Geometry: final body of the model. Coordinates: model frame, mm. Give positions to 0.01 mm unless a question says otherwise; leave off trailing zeros. Loops run counter-clockwise (first coordinate to the right, second up) from the corner with the lowest first, then second, coordinate; pieces in that order, holes last. Notation, with made-up numbers: (-39.75, 8.5) - (14.25, 8.5) arc R25 ccw to (14.25, 45.5) - close; hole circle Ø1 at (43.25, 5.5). An arc over 180 degrees is marked (long way). Answer in a Markdown table with one row per item.
from build123d import *

# Parameters (mm, degrees)
SKETCH_1_W      = 110
SKETCH_1_H      = 116
SKETCH_1_R      = 4.5
SKETCH_1_R_2    = 2
EXTRUDE_1_DEPTH = 14
FILLET_1_R      = 3


with BuildPart() as part:
    # 草图1 → 凸台-拉伸1 (new body)
    with BuildSketch(Plane(origin=(0, 0, 0), x_dir=(1, 0, 0), z_dir=(0, 1, 0))):
        Rectangle(SKETCH_1_W, SKETCH_1_H)
        with Locations(Location((-43, 30, 0), (0, 0, 270))):
            Circle(SKETCH_1_R, mode=Mode.SUBTRACT)
        with Locations(Location((43, 30, 0), (0, 0, 270))):
            Circle(SKETCH_1_R, mode=Mode.SUBTRACT)
        with Locations(Location((43, -30, 0), (0, 0, 270))):
            Circle(SKETCH_1_R, mode=Mode.SUBTRACT)
        with Locations(Location((-43, -30, 0), (0, 0, 270))):
            Circle(SKETCH_1_R, mode=Mode.SUBTRACT)
        with Locations(Location((0, -50, 0), (0, 0, 270))):
            Circle(SKETCH_1_R_2, mode=Mode.SUBTRACT)
        with Locations(Location((0, 50, 0), (0, 0, 90))):
            Circle(SKETCH_1_R_2, mode=Mode.SUBTRACT)
    extrude(amount=EXTRUDE_1_DEPTH)

    # 圆角1
    fillet_1_edges = [part.edges().sort_by_distance(p)[0] for p in [
        (-55, 7, -58),
        (55, 7, -58),
        (55, 7, 58),
        (-55, 7, 58),
    ]]
    fillet(fillet_1_edges, radius=FILLET_1_R)


solid = part.part
Q1. Cut plane A-A (z = 30). Output: boundary loops of the cut face in (x, y), and give its area (3 significant figures).
Check values:
| item | result |
|---|---|
| outline | (-55, 0) - (-47.5, 0) - (-47.5, 14) - (-55, 14) - close; (-38.5, 0) - (38.5, 0) - (38.5, 14) - (-38.5, 14) - close; (47.5, 0) - (55, 0) - (55, 14) - (47.5, 14) - close |
| area | 1,290 mm² |
Q2. Cut plane D-D (z = -50). Output: boundary loops of the cut face in (x, y).
Check values:
| item | result |
|---|---|
| outline | (-55, 0) - (-2, 0) - (-2, 14) - (-55, 14) - close; (2, 0) - (55, 0) - (55, 14) - (2, 14) - close |
Q3. Material intervals for line 1 along X through (y, z) = (6.75, 30); line 2 along Z through (x, y) = (-41.5, 7); line 3 along X through (y, z) = (9.75, 50), sorted ascending.
Check values:
| item | result |
|---|---|
| line 1 | -55 to -47.5, -38.5 to 38.5, 47.5 to 55 |
| line 2 | -58 to -34.24, -25.76 to 25.76, 34.24 to 58 |
| line 3 | -55 to -2, 2 to 55 |
Q4. Draft query along Z for faces 1 (the cylindrical face through (-0.766, 6.902, 51.847)), 2 (the flat face through (-1, 7, 58)), 3 (the cylindrical face through (54.1, 7.1, -57.14)). Return one class per face: pulls with the +Z half, pulls with the -Z half, needs draft (parallel to the pull), parting line crosses it, or undercut.
Check values:
| item | result |
|---|---|
| face 1 | undercut |
| face 2 | pulls with the +Z half |
| face 3 | pulls with the -Z half |
Q5. Cut plane B-B (x = -43). Output: boundary loops of the cut face in (y, z), and give its area (3 significant figures).
Check values:
| item | result |
|---|---|
| outline | (0, -58) - (14, -58) - (14, -34.5) - (0, -34.5) - close; (0, -25.5) - (14, -25.5) - (14, 25.5) - (0, 25.5) - close; (0, 34.5) - (14, 34.5) - (14, 58) - (0, 58) - close |
| area | 1,370 mm² |
Q6. Cut plane C-C (y = 9.25). Output: boundary loops of the cut face in (x, z), and give its area (3 significant figures).
Check values:
| item | result |
|---|---|
| outline | (-55, -55) arc R3 ccw to (-52, -58) - (52, -58) arc R3 ccw to (55, -55) - (55, 55) arc R3 ccw to (52, 58) - (-52, 58) arc R3 ccw to (-55, 55) - close; hole circle Ø9 at (-43, -30); hole circle Ø9 at (-43, 30); hole circle Ø4 at (0, -50); hole circle Ø4 at (0, 50); hole circle Ø9 at (43, -30); hole circle Ø9 at (43, 30) |
| area | 12,500 mm² |
